Could you check a few things on this model? Use its own coordinates, in mm. Face numbers are marked on the shaded views. Round coordinates to 2 decimals unless told otherwise and drop trailing zeros. Order: outer loops, then holes, each group sorted by start corner. A loop starts at its lowest first (then second) coordinate and runs counter-clockwise, first axis right, second up. Notation, with made-up numbers: M 25.25,60.5 L 31.25,60.5 A32 cw 31.25,89.5 Z; hole C -2.5,50 d3. An arc over 180 degrees is marked long. Write each question's results on one line, items separated by ' | '. Start each with the question number.
1. We'd pull the mould along X, two halves only. Please class the marked faces 1, 2, 3 and 4: released by +X, released by -X, zero draft, split by the parting line, or undercut.
2. Please list where these lines run through material, in increasing order: L1, parallel to X at y = -16.5, z = 28; L2, parallel to X at y = -30.4, z = 16; L3, parallel to Y at x = -7, z = 57.5.
3. Suppose I cut it at C-C on z = 155. Write out the boundary of the cut face in (x, y).
4. Suppose I cut it at B-B on y = -8.5. Write out the boundary of the cut face in (x, z).
5. Suppose I cut it at D-D on z = 25. Write out the boundary of the cut face in (x, y), and give its area (3 significant figures).
6. I'm going to push flat-ended pins straight in: pin 1 (1.5 mm diameter, centred on x = 4, y = -31, fed in from +Z); pin 2 (3 mm diameter, centred on x = 19.5, z = 34, fed in from +Y); pin 3 (2.5 mm diameter, centred on y = -31, z = 13.5, fed in from -X). Where does each tip first touch, or does it pass through?
7. Suppose I cut it at A-A on z = 56. Write out the boundary of the cut face in (x, y).
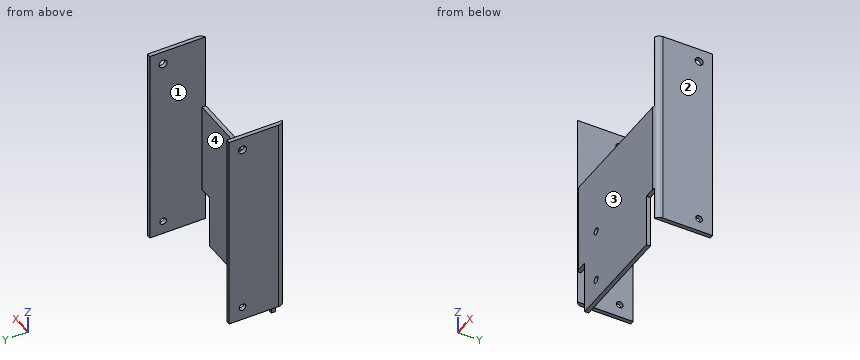
from build123d import *

# Parameters (mm, degrees)
SALIENTE_EXTRUIR1_DEPTH = 165
CROQUIS3_W              = 10
CROQUIS3_H              = 40
CORTAR_EXTRUIR1_DEPTH   = 165
CROQUIS4_W              = 3
CROQUIS4_H              = 15
CORTAR_EXTRUIR2_DEPTH   = 165
CROQUIS5_W              = 101
CROQUIS5_H              = 57
CORTAR_EXTRUIR3_DEPTH   = 165
CROQUIS6_R              = 2.5
CORTAR_EXTRUIR4_DEPTH   = 165
REDONDEO1_R             = 5
CROQUIS7_R              = 3
CORTAR_EXTRUIR5_DEPTH   = 110
CROQUIS8_R              = 2.5
CORTAR_EXTRUIR6_DEPTH   = 10


with BuildPart() as part:
    # Croquis2 → Saliente-Extruir1 (new body)
    with BuildSketch(Plane.XY):
        Polygon((61.739775044, 10), (61.739775044, -32), (-45.260224956, -32), (-45.260224956, 10), (-42.260224956, 10), (-42.260224956, -29), (58.739775044, -29), (58.739775044, 10), align=None)
    extrude(amount=SALIENTE_EXTRUIR1_DEPTH)

    # Croquis3 → Cortar-Extruir1 (cut)
    with BuildSketch(Plane(origin=(0, -29, 0), x_dir=(1, 0, 0), z_dir=(0, 1, 0))):
        with Locations((-37.260224956, -20)):
            Rectangle(CROQUIS3_W, CROQUIS3_H)
        with Locations((53.739775044, -20)):
            Rectangle(CROQUIS3_W, CROQUIS3_H)
    extrude(amount=-CORTAR_EXTRUIR1_DEPTH, mode=Mode.SUBTRACT)

    # Croquis4 → Cortar-Extruir2 (cut)
    with BuildSketch(Plane(origin=(0, 10, 0), x_dir=(1, 0, 0), z_dir=(0, 1, 0))):
        with Locations((-43.760224956, -7.5)):
            Rectangle(CROQUIS4_W, CROQUIS4_H)
        with Locations((60.239775044, -7.5)):
            Rectangle(CROQUIS4_W, CROQUIS4_H)
    extrude(amount=-CORTAR_EXTRUIR2_DEPTH, mode=Mode.SUBTRACT)

    # Croquis5 → Cortar-Extruir3 (cut)
    with BuildSketch(Plane(origin=(0, -29, 0), x_dir=(1, 0, 0), z_dir=(0, 1, 0))):
        with Locations((8.239775044, -136.5)):
            Rectangle(CROQUIS5_W, CROQUIS5_H)
    extrude(amount=-CORTAR_EXTRUIR3_DEPTH, mode=Mode.SUBTRACT)

    # Croquis6 → Cortar-Extruir4 (cut)
    with BuildSketch(Plane(origin=(61.739775044, 0, 0), x_dir=(0, 0, -1), z_dir=(1, 0, 0))):
        with Locations((-25, 0)):
            Circle(CROQUIS6_R)
        with Locations((-155, 0)):
            Circle(CROQUIS6_R)
    extrude(amount=-CORTAR_EXTRUIR4_DEPTH, mode=Mode.SUBTRACT)

    # Redondeo1
    redondeo1_edges = [part.edges().sort_by_distance(p)[0] for p in [
        (61.739775044, -32, 90),
        (-45.260224956, -32, 90),
    ]]
    fillet(redondeo1_edges, radius=REDONDEO1_R)

    # Croquis7 → Cortar-Extruir5 (cut)
    with BuildSketch(Plane(origin=(61.739775044, 0, 0), x_dir=(0, 0, -1), z_dir=(1, 0, 0))):
        with Locations((-155, 0)):
            Circle(CROQUIS7_R)
    extrude(amount=-CORTAR_EXTRUIR5_DEPTH, mode=Mode.SUBTRACT)

    # Croquis8 → Cortar-Extruir6 (cut)
    with BuildSketch(Plane(origin=(0, -29, 0), x_dir=(1, 0, 0), z_dir=(0, 1, 0))):
        with Locations((-17.260224956, -16)):
            Circle(CROQUIS8_R)
        with Locations((-17.260224956, -56)):
            Circle(CROQUIS8_R)
    extrude(amount=-CORTAR_EXTRUIR6_DEPTH, mode=Mode.SUBTRACT)


solid = part.part
Filled sheet:
1) face 1: undercut | face 2: released by +X | face 3: zero draft | face 4: undercut
2) L1: x = -45.26 to -42.26, 58.74 to 61.74 | L2: x = -43.93 to -42.26, -32.26 to -19.76, -14.76 to 48.74, 58.74 to 60.41 | L3: y = -32 to -29
3) outline: M -45.26,-27 A5 ccw -42.26,-31.58 L -42.26,-3 L -45.26,-3 Z; M -45.26,3 L -42.26,3 L -42.26,10 L -45.26,10 Z; M 58.74,-31.58 A5 ccw 61.74,-27 L 61.74,-3 L 58.74,-3 Z; M 58.74,3 L 61.74,3 L 61.74,10 L 58.74,10 Z
4) outline: M -45.26,15 L -42.26,15 L -42.26,165 L -45.26,165 Z; M 58.74,15 L 61.74,15 L 61.74,165 L 58.74,165 Z
5) outline: M -45.26,-27 A5 ccw -42.26,-31.58 L -42.26,-2.5 L -45.26,-2.5 Z; M -45.26,2.5 L -42.26,2.5 L -42.26,10 L -45.26,10 Z; M -32.26,-32 L 48.74,-32 L 48.74,-29 L -32.26,-29 Z; M 58.74,-31.58 A5 ccw 61.74,-27 L 61.74,-2.5 L 58.74,-2.5 Z; M 58.74,2.5 L 61.74,2.5 L 61.74,10 L 58.74,10 Z | area: 455 mm^2
6) pin 1: stops at z = 108 | pin 2: stops at y = -29 | pin 3: stops at x = -32.26
7) outline: M -45.26,-27 A5 ccw -40.26,-32 L -19.76,-32 L -19.76,-29 L -42.26,-29 L -42.26,10 L -45.26,10 Z; M -14.76,-32 L 56.74,-32 A5 ccw 61.74,-27 L 61.74,10 L 58.74,10 L 58.74,-29 L -14.76,-29 Z
